Input: part model. Units: mm. Frame: model coordinates. Face numbers are marked on the shaded views. A direction names the side the tool comes from. Round coordinates to 2 decimals unless told otherwise and drop trailing zeros. Write each loop counter-clockwise with the first axis right and the second up, starting at its lowest first coordinate (ties: lowest second). Pieces come first, ordered by that corner, then holes. Notation, with made-up numbers: (4, 5) -> (57, 5) arc R31 ccw to (57, 30) -> close; hole circle Ø2 at (0.5, -18). An arc over 180 degrees is marked (long way). Write item = value, one per line.
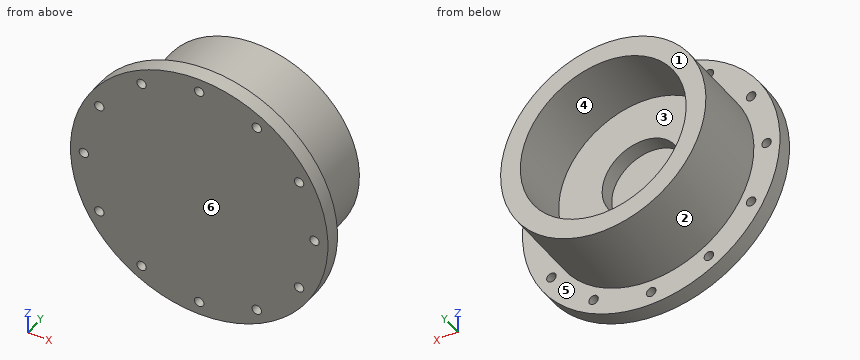
```python
from build123d import *

# Parameters (mm, degrees)
BOSS_EXTRUDE1_START = -20
SKETCH2_R           = 81.5
SKETCH2_R_2         = 3
BOSS_EXTRUDE1_DEPTH = 10


with BuildPart() as part:
    # Sketch1 → Revolve1 (revolve)
    with BuildSketch(Plane(origin=(0, 0, 0), x_dir=(0, 0, -1), z_dir=(1, 0, 0))):
        Polygon((25, 0), (25, -10), (0, -10), (0, -20), (65, -20), (65, -10), (65, 40), (52.5, 40), (52.5, 0), align=None)
    revolve(axis=Axis((0, 0, 0), (0, 1, 0)))

    # Sketch2 → Boss-Extrude1 (add)
    with BuildSketch(Plane(origin=(0, 0, 0), x_dir=(1, 0, 0), z_dir=(0, 1, 0)).offset(BOSS_EXTRUDE1_START)):
        with Locations(Location((0, 0, 0), (0, 0, 90))):
            Circle(SKETCH2_R)
        with Locations(Location((0, 73, 0), (0, 0, 90))):
            Circle(SKETCH2_R_2, mode=Mode.SUBTRACT)
        with Locations(Location((36.5, 63.219854476, 0), (0, 0, 90))):
            Circle(SKETCH2_R_2, mode=Mode.SUBTRACT)
        with Locations(Location((63.219854476, 36.5, 0), (0, 0, 90))):
            Circle(SKETCH2_R_2, mode=Mode.SUBTRACT)
        with Locations(Location((73, 0, 0), (0, 0, 90))):
            Circle(SKETCH2_R_2, mode=Mode.SUBTRACT)
        with Locations(Location((63.219854476, -36.5, 0), (0, 0, 90))):
            Circle(SKETCH2_R_2, mode=Mode.SUBTRACT)
        with Locations(Location((36.5, -63.219854476, 0), (0, 0, 90))):
            Circle(SKETCH2_R_2, mode=Mode.SUBTRACT)
        with Locations(Location((0, -73, 0), (0, 0, 90))):
            Circle(SKETCH2_R_2, mode=Mode.SUBTRACT)
        with Locations(Location((-36.5, -63.219854476, 0), (0, 0, 90))):
            Circle(SKETCH2_R_2, mode=Mode.SUBTRACT)
        with Locations(Location((-63.219854476, -36.5, 0), (0, 0, 90))):
            Circle(SKETCH2_R_2, mode=Mode.SUBTRACT)
        with Locations(Location((-73, 0, 0), (0, 0, 90))):
            Circle(SKETCH2_R_2, mode=Mode.SUBTRACT)
        with Locations(Location((-63.219854476, 36.5, 0), (0, 0, 90))):
            Circle(SKETCH2_R_2, mode=Mode.SUBTRACT)
        with Locations(Location((-36.5, 63.219854476, 0), (0, 0, 90))):
            Circle(SKETCH2_R_2, mode=Mode.SUBTRACT)
    extrude(amount=BOSS_EXTRUDE1_DEPTH)


solid = part.part
```
1) Access query for the marked faces 5 and 6. Directions: +Z, -Z, +X, -X, +Y, -Y. A direction counts if a zero-diameter tool reaches every point of the face in a straight line with its end or side. Return the directions, or none.
Solutions:
face_5 = +Y
face_6 = +Z, -Z, +X, -X, -Y
2) Cut plane D-D (y = -15.5). Count the separate pieces of the cut face and the enclosed holes in it, and give its area (3 significant figures).
Solutions:
separate_pieces = 1
enclosed_holes = 12
area = 20,500 mm^2
3) Cut plane C-C (z = 73). Return the cut outline in (x, y), and give its area (3 significant figures).
Solutions:
outline = (-36.24, -20) -> (-3, -20) -> (-3, -10) -> (-36.24, -10) -> close; (3, -20) -> (36.24, -20) -> (36.24, -10) -> (3, -10) -> close
area = 665 mm^2
4) First-contact query: P1, Ø12, axis at x = -34.5, y = -7.5, coming from the -Z side; P2, Ø8, axis at y = 31, z = 9.5, coming from the +X side; P3, Ø1, axis at x = -45.5, y = 11.5, coming from the +Z side; P4, Ø5, axis at x = -63.22, z = 36.5, coming from the -Y side. Flat tips, straight axial feed; report the tip coordinate or a pass-through.
Solutions:
P1 = -76.15
P2 = 64.77
P3 = 46.9
P4 = through
5) Draft query along Z for the marked faces 1, 2, 3 and 4. Return one class per face: +Z half, -Z half, draft (parallel to the pull), parting line (faces both ways), or undercut.
Solutions:
face_1 = draft
face_2 = parting line
face_3 = undercut
face_4 = undercut
6) Line query: L1, parallel to X at y = -9.5, z = 0.5 (3 decimals); L2, parallel to X at y = 29, z = 0; L3, parallel to Z at x = -22, y = 2.5. Output: solid intervals per line, ascending. Write a range as from..to.
Solutions:
L1 = -64.998..-24.995, 24.995..64.998
L2 = -65..-52.5, 52.5..65
L3 = -61.16..-47.67, 47.67..61.16
7) Cut plane A-A (z = 0). Return the cut outline in (x, y).
Solutions:
outline = (-81.5, -20) -> (-76, -20) -> (-76, -10) -> (-81.5, -10) -> close; (-70, -20) -> (70, -20) -> (70, -10) -> (65, -10) -> (65, 40) -> (52.5, 40) -> (52.5, 0) -> (25, 0) -> (25, -10) -> (-25, -10) -> (-25, 0) -> (-52.5, 0) -> (-52.5, 40) -> (-65, 40) -> (-65, -10) -> (-70, -10) -> close; (76, -20) -> (81.5, -20) -> (81.5, -10) -> (76, -10) -> close
8) Cut plane B-B (x = 0). Return the cut outline in (y, z).
Solutions:
outline = (-20, -81.5) -> (-10, -81.5) -> (-10, -76) -> (-20, -76) -> close; (-20, -70) -> (-10, -70) -> (-10, -65) -> (40, -65) -> (40, -52.5) -> (0, -52.5) -> (0, -25) -> (-10, -25) -> (-10, 25) -> (0, 25) -> (0, 52.5) -> (40, 52.5) -> (40, 65) -> (-10, 65) -> (-10, 70) -> (-20, 70) -> close; (-20, 76) -> (-10, 76) -> (-10, 81.5) -> (-20, 81.5) -> close
